```python
from build123d import *

# Parameters (mm, degrees)
SKETCH_1_W      = 25
SKETCH_1_H      = 25
SKETCH_1_R      = 1.5
EXTRUDE_1_DEPTH = 1


with BuildPart() as part:
    # 草图1 → 凸台-拉伸1 (new body)
    with BuildSketch(Plane.XY):
        Rectangle(SKETCH_1_W, SKETCH_1_H)
        with Locations((9.5, -9.5)):
            Circle(SKETCH_1_R, mode=Mode.SUBTRACT)
        with Locations(Location((-9.5, -9.5, 0), (0, 0, 180))):
            Circle(SKETCH_1_R, mode=Mode.SUBTRACT)
        with Locations((0, 6.954482672)):
            Circle(SKETCH_1_R, mode=Mode.SUBTRACT)
    extrude(amount=EXTRUDE_1_DEPTH)


solid = part.part
```
Geometry check sheet. Reference: the model listing, model coordinates, mm. Coordinates: 2 decimals unless noted, no trailing zeros. Order: outer loops, then holes, each group sorted by start corner. A loop starts at its lowest first (then second) coordinate and runs counter-clockwise, first axis right, second up.
Item 1: Section check D-D (y = 5.75). Enter the section's corners in (x, z).
Item 2: Scan lines: line 1 along Y through (x, z) = (-9.5, 0.5); line 2 along X through (y, z) = (-9.75, 0.7); line 3 along Y through (x, z) = (0, 0.5). Record each from-to range of solid material in increasing order.
Item 3: Section check A-A (y = -9.5). Enter the section's corners in (x, z), plus the area to 3 significant figures.
Item 4: Mould release check, pull along Y, two halves, no side actions. Record for faces 1 (the flat face through (-0.2, 12.5, 0.5)), 2 (the flat face through (0, 0, 0)), 3 (the cylindrical face through (8.3, -10.4, 0.5)): released by +Y, released by -Y, zero draft, split by the parting line, or undercut.
Item 5: Section check B-B (x = -9.5). Enter the section's corners in (y, z), plus the area to 3 significant figures.
Item 6: Depth check by flat-ended pin: pin 1 (2.5 mm diameter, centred on x = 9.5, y = -9.5, fed in from +Z). Enter the tip coordinate at first touch or a pass-through.
Item 7: Section check C-C (z = 0.7). Enter the section's corners in (x, y).
Check sheet entries:
1. outline: (-12.5, 0) - (-0.89, 0) - (-0.89, 1) - (-12.5, 1) - close; (0.89, 0) - (12.5, 0) - (12.5, 1) - (0.89, 1) - close
2. line 1: y = -12.5 to -11, -8 to 12.5
2. line 2: x = -12.5 to -10.98, -8.02 to 8.02, 10.98 to 12.5
2. line 3: y = -12.5 to 5.45, 8.45 to 12.5
3. outline: (-12.5, 0) - (-11, 0) - (-11, 1) - (-12.5, 1) - close; (-8, 0) - (8, 0) - (8, 1) - (-8, 1) - close; (11, 0) - (12.5, 0) - (12.5, 1) - (11, 1) - close
3. area: 19.0 mm2
4. face 1: released by +Y
4. face 2: zero draft
4. face 3: undercut
5. outline: (-12.5, 0) - (-11, 0) - (-11, 1) - (-12.5, 1) - close; (-8, 0) - (12.5, 0) - (12.5, 1) - (-8, 1) - close
5. area: 22.0 mm2
6. pin 1: passes through
7. outline: (-12.5, -12.5) - (12.5, -12.5) - (12.5, 12.5) - (-12.5, 12.5) - close; hole circle Ø3 at (-9.5, -9.5); hole circle Ø3 at (0, 6.95); hole circle Ø3 at (9.5, -9.5)
